Input: dimensioned drawing with shaded views. Units: mm. Origin: part minimum x, y, z. A direction names the side the tool comes from. Round coordinates to 2 decimals unless told otherwise and drop trailing zeros. Loops run counter-clockwise (first coordinate to the right, second up) from the corner with the lowest first, then second, coordinate; pieces in that order, holes last. Notation, with made-up numbers: M -3,24 L 1,24 A28 ccw 1,50 Z; hole C 42,39.5 d2. An arc over 180 degrees is marked long. Write each question's results on one line, items separated by ' | '. Start each with the question number.
1. Section A-A on z = 0.5. Output: boundary loops of the cut face in (x, y) (3 decimals), and give its area (4 significant figures).
2. Contact query for flat-ended pins moving along their axis: pin 1 Ø3 at (x, y) = (4, 13) entering from +Z; pin 2 Ø1.5 at (x, z) = (1, 2) entering from +Y; pin 3 Ø2 at (y, z) = (14.5, 1) entering from +X (3 decimals). Output: stop coordinate, or through.
3. Section C-C on x = 1.75. Output: boundary loops of the cut face in (y, z), and give its area (3 significant figures).
4. Ray query, line 1 (Y direction, x = 2.5, z = 1.05); line 2 (X direction, y = 5.75, z = 2) (3 decimals); line 3 (Z direction, x = 3, y = 22). Return the intervals inside material, ascending.
5. Section B-B on y = 15.5. Output: boundary loops of the cut face in (x, z) (3 decimals).
6. Set-up query: the marked faces 1, 2, 3, 4 and 5. Return all of +Z, -Z, +X, -X, +Y, -Y with unobstructed straight access to the full face (end or side cutting, diameter ignored); none if empty.
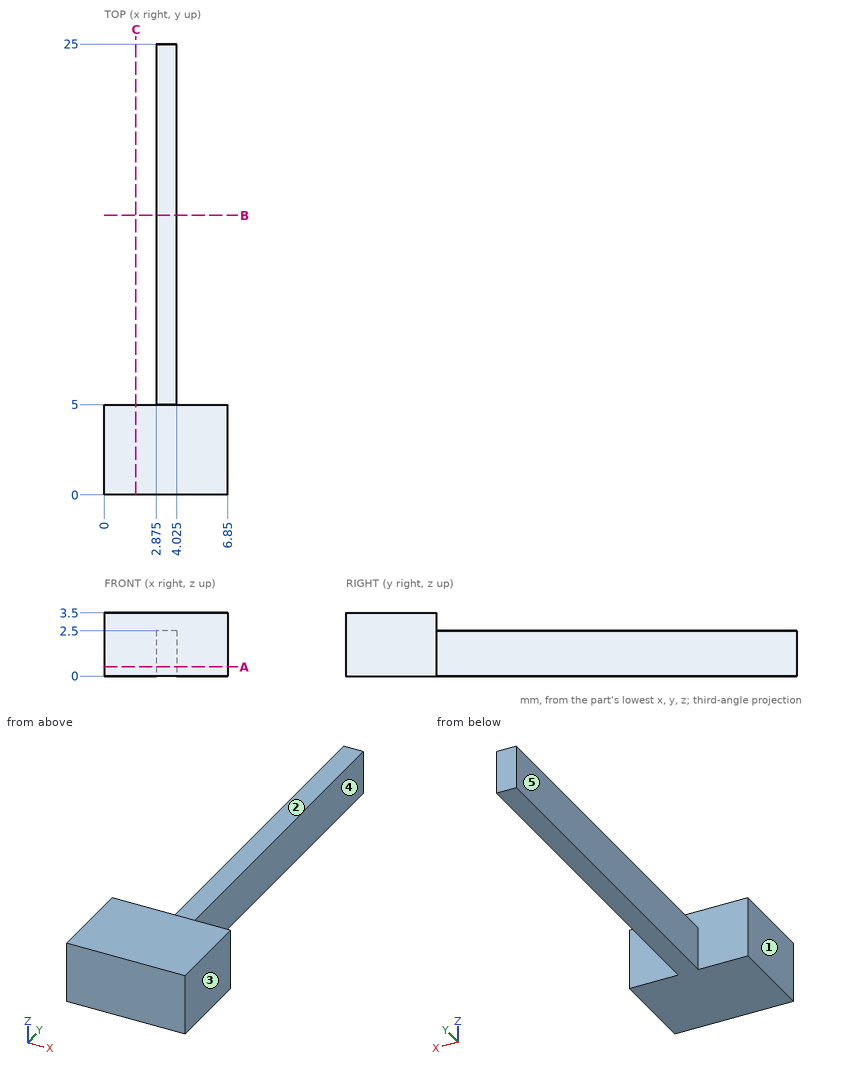
Taken from the geometry:
1) outline: M 0,0 L 6.85,0 L 6.85,5 L 4.025,5 L 4.025,25 L 2.875,25 L 2.875,5 L 0,5 Z | area: 57.25 mm^2
2) pin 1: z = 2.5 | pin 2: y = 5 | pin 3: x = 4.025
3) outline: M 0,0 L 5,0 L 5,3.5 L 0,3.5 Z | area: 17.5 mm^2
4) line 1: 0 to 5 | line 2: 2.875 to 4.025 | line 3: 0 to 2.5
5) outline: M 2.875,0 L 4.025,0 L 4.025,2.5 L 2.875,2.5 Z
6) face 1: +Z, -Z, -X, +Y, -Y | face 2: +Z, +X, -X, +Y | face 3: +Z, -Z, +X, +Y, -Y | face 4: +Z, -Z, +X, +Y | face 5: +Z, -Z, -X, +Y
